from build123d import *

# Parameters (mm, degrees)
SKETCH1_W           = 50.8
SKETCH1_H           = 35.4
SKETCH1_R           = 3.5
BOSS_EXTRUDE1_DEPTH = 5
SKETCH2_W           = 50.8
SKETCH2_H           = 45
BOSS_EXTRUDE2_DEPTH = 5
SKETCH3_R           = 1.7
CUT_EXTRUDE1_DEPTH  = 5
BOSS_EXTRUDE3_DEPTH = 2.5
BOSS_EXTRUDE4_DEPTH = 2.5


with BuildPart() as part:
    # Sketch1 → Boss-Extrude1 (new body)
    with BuildSketch(Plane(origin=(0, 0, 0), x_dir=(1, 0, 0), z_dir=(0, 1, 0))):
        with Locations((-25.4, 17.7)):
            Rectangle(SKETCH1_W, SKETCH1_H)
        with Locations((-38.1, 12.7)):
            Circle(SKETCH1_R, mode=Mode.SUBTRACT)
        with Locations((-12.7, 12.7)):
            Circle(SKETCH1_R, mode=Mode.SUBTRACT)
    extrude(amount=BOSS_EXTRUDE1_DEPTH)

    # Sketch2 → Boss-Extrude2 (add)
    with BuildSketch(Plane(origin=(0, 0, -35.4), x_dir=(-1, 0, 0), z_dir=(0, 0, -1))):
        with Locations((25.4, 22.5)):
            Rectangle(SKETCH2_W, SKETCH2_H)
    extrude(amount=BOSS_EXTRUDE2_DEPTH)

    # Sketch3 → Cut-Extrude1 (cut)
    with BuildSketch(Plane(origin=(0, 0, -40.4), x_dir=(-1, 0, 0), z_dir=(0, 0, -1))):
        with Locations((25.4, 33.75)):
            Circle(SKETCH3_R)
    extrude(amount=-CUT_EXTRUDE1_DEPTH, mode=Mode.SUBTRACT)

    # Sketch4 → Boss-Extrude3 (add)
    with BuildSketch(Plane(origin=(0, 0, 0), x_dir=(0, 0, -1), z_dir=(1, 0, 0))):
        Polygon((0, 5), (35.4, 45), (40.4, 45), (40.4, 0), (0, 0), align=None)
    extrude(amount=-BOSS_EXTRUDE3_DEPTH)

    # Sketch5 → Boss-Extrude4 (add)
    with BuildSketch(Plane.ZY.offset(50.8)):
        Polygon((-35.4, 45), (-40.4, 45), (-40.4, 0), (0, 0), (0, 5), align=None)
    extrude(amount=BOSS_EXTRUDE4_DEPTH)


solid = part.part
The listing builds one solid part. Answer for the finished solid, in the listing's coordinates (mm). A direction names the side the tool comes from. Coordinates: 2 decimals unless noted, no trailing zeros. Loops run counter-clockwise (first coordinate to the right, second up) from the corner with the lowest first, then second, coordinate; pieces in that order, holes last. Notation, with made-up numbers: (41.5, -17.5) -> (69.5, -17.5) arc R13 cw to (69.5, -12.5) -> close; hole circle Ø10 at (-25, 29.25). An arc over 180 degrees is marked (long way). Write item = value, one per line. Start each with the question number.
1) Straight lines are drawn through the part: line 1 (X direction, y = 2, z = -12.7); line 2 (X direction, y = 2, z = -12); line 3 (Z direction, x = -38.1, y = 3.6). For each, find the intervals that lie inside material, in ascending order. Write a range as from..to.
2) A cutting plane is placed at D-D (x = -25.4). Give the vertices of the cut face in (y, z), then the cut area to 3 significant figures.
3) A cutting plane is placed at A-A (x = -38.1). Give the vertices of the cut face in (y, z).
4) The mould has two halves that part along Z. Classify faces 1 (the face through (-52.03, 24.72, -17.45)), 2 (the face through (-34.76, 2.46, -13.75)), 3 (the face through (-50.8, 16, -26)), 4 (the face through (-10.82, 2.46, -15.65)): released by +Z, released by -Z, zero draft, split by the parting line, or undercut.
5) A cutting plane is placed at B-B (z = -12). Give the vertices of the cut face in (x, y), then the cut area to 3 significant figures.
6) A cutting plane is placed at C-C (y = 33.75). Give the vertices of the cut face in (x, z).
7) Given pin 1 Ø5 at (x, z) = (-25, -20.5) entering from +Y; pin 2 Ø20 at (x, y) = (-38.5, 24) entering from +Z, each flat-ended and moving along its own axis, determine where each tip first touches the part or whether it passes through.
8) A tool of negligible diameter and unlimited length cuts with its end or side. For faces 5 (the face through (-26, 23, -40.4)), 6 (the face through (-2.5, 16, -26)), from which of +Z, -Z, +X, -X, +Y, -Y can it reach the whole face along a straight path? Write none if from no direction.
Responses:
q1.line_1 = -53.3..-41.6, -34.6..-16.2, -9.2..0
q1.line_2 = -53.3..-41.53, -34.67..-16.13, -9.27..0
q1.line_3 = -40.4..-16.2, -9.2..0
q2.outline = (0, -40.4) -> (32.05, -40.4) -> (32.05, -35.4) -> (5, -35.4) -> (5, 0) -> (0, 0) -> close; (35.45, -40.4) -> (45, -40.4) -> (45, -35.4) -> (35.45, -35.4) -> close
q2.area = 385 mm²
q3.outline = (0, -40.4) -> (45, -40.4) -> (45, -35.4) -> (5, -35.4) -> (5, -16.2) -> (0, -16.2) -> close; (0, -9.2) -> (5, -9.2) -> (5, 0) -> (0, 0) -> close
q4.face_1 = released by +Z
q4.face_2 = undercut
q4.face_3 = zero draft
q4.face_4 = undercut
q5.outline = (-53.3, 0) -> (-41.53, 0) -> (-41.53, 5) -> (-50.8, 5) -> (-50.8, 18.56) -> (-53.3, 18.56) -> close; (-34.67, 0) -> (-16.13, 0) -> (-16.13, 5) -> (-34.67, 5) -> close; (-9.27, 0) -> (0, 0) -> (0, 18.56) -> (-2.5, 18.56) -> (-2.5, 5) -> (-9.27, 5) -> close
q5.area = 266 mm²
q6.outline = (-53.3, -40.4) -> (-27.1, -40.4) -> (-27.1, -35.4) -> (-50.8, -35.4) -> (-50.8, -25.44) -> (-53.3, -25.44) -> close; (-23.7, -40.4) -> (0, -40.4) -> (0, -25.44) -> (-2.5, -25.44) -> (-2.5, -35.4) -> (-23.7, -35.4) -> close
q7.pin_1 = 5
q7.pin_2 = -35.4
q8.face_5 = -Z, +X, -X, +Y, -Y
q8.face_6 = +Z, +Y
